Part model, mm, in its own coordinate system. Give positions to 0.01 mm unless a question says otherwise; leave off trailing zeros. Write each loop counter-clockwise with the first axis right and the second up, starting at its lowest first coordinate (ties: lowest second). Pieces come first, ordered by that corner, then holes. Notation, with made-up numbers: (6, -36.75) - (35, -36.75) arc R21 cw to (35, -7.75) - close; hole circle Ø5 at (50.25, -3). An arc over 180 degrees is marked (long way). Answer as a JSON object with one key per item and string values. Group by question number.
```python
from build123d import *

# Parameters (mm, degrees)
SKETCH1_R           = 4.445
SKETCH1_W           = 3.175
SKETCH1_H           = 12.7
SKETCH1_H_2         = 3.175
SKETCH1_W_2         = 25.4
BOSS_EXTRUDE1_DEPTH = 3.175


with BuildPart() as part:
    # Sketch1 → Boss-Extrude1 (new body)
    with BuildSketch(Plane.XY):
        with BuildLine():
            ThreePointArc((-23.00901311, 85.870805957), (0, -88.9), (23.00901311, 85.870805957))
            add(Edge.make_bspline(
                [(23.00901311, 85.870805957), (14.830841114, 88.062140539), (8.89, 90.527472624), (8.89, 94.760805957)],
                knots=[0, 0, 0, 0, 1, 1, 1, 1], degree=3))
            ThreePointArc((8.89, 94.760805957), (0, 103.650805957), (-8.89, 94.760805957))
            add(Edge.make_bspline(
                [(-23.00901311, 85.870805957), (-14.830841114, 88.062140539), (-8.89, 90.527472624), (-8.89, 94.760805957)],
                knots=[0, 0, 0, 0, 1, 1, 1, 1], degree=3))
        make_face()
        with Locations((0, 94.760805957)):
            Circle(SKETCH1_R, mode=Mode.SUBTRACT)
        with Locations((77.7875, 25.38476)):
            Rectangle(SKETCH1_W, SKETCH1_H, mode=Mode.SUBTRACT)
        Rectangle(SKETCH1_W, SKETCH1_H_2, mode=Mode.SUBTRACT)
        with Locations((77.7875, -25.41524)):
            Rectangle(SKETCH1_W, SKETCH1_H, mode=Mode.SUBTRACT)
        with Locations((-77.7875, -25.41524)):
            Rectangle(SKETCH1_W, SKETCH1_H, mode=Mode.SUBTRACT)
        with Locations((-77.7875, 25.38476)):
            Rectangle(SKETCH1_W, SKETCH1_H, mode=Mode.SUBTRACT)
        with Locations((0, 80.9625)):
            Rectangle(SKETCH1_W_2, SKETCH1_H_2, mode=Mode.SUBTRACT)
        with Locations((0, -80.9625)):
            Rectangle(SKETCH1_W_2, SKETCH1_H_2, mode=Mode.SUBTRACT)
    extrude(amount=BOSS_EXTRUDE1_DEPTH)


solid = part.part
```
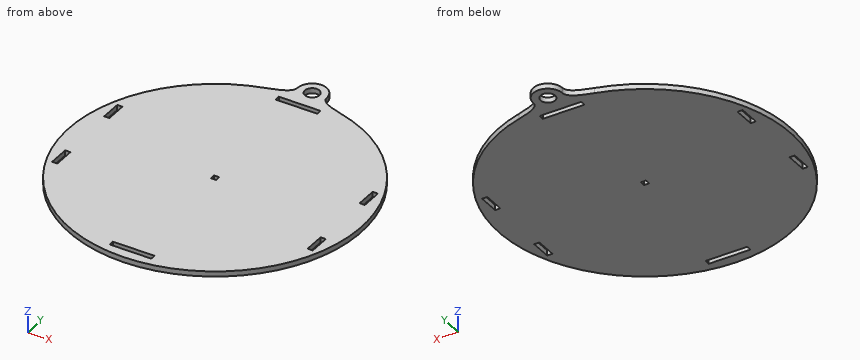
1) Band-saw the part on B-B (z = 1.15). State how many separate pieces and enclosed holes the cut face has, plus the area to 3 significant figures.
2) Drop flat-ended pins along their axis: P1, Ø1.6, axis at y = 81.5, z = 1.5, coming from the +X side; P2, Ø1, axis at y = 23, z = 1, coming from the -X side; P3, Ø1.5, axis at y = 46.5, z = 2.5, coming from the -X side. Give the stop position or say it passes through.
3) Probe line 1 (X direction, y = -19.5, z = 1.8) (3 decimals); line 2 (X direction, y = 26, z = 1.85) (3 decimals); line 3 (X direction, y = -33, z = 0.9). List the from-to ranges inside material, lowest first.
4) Band-saw the part on C-C (y = -46). List the corners of the cut face in (x, z) (3 decimals).
5) Band-saw the part on A-A (y = -24). List the corners of the cut face in (x, z) (3 decimals).
6) Band-saw the part on D-D (x = -43). List the corners of the cut face in (y, z) (3 decimals).
Verdict:
{
 "1": {"separate pieces": "1", "enclosed holes": "8", "area": "24,700 mm2"},
 "2": {"P1": "x = 37.29", "P2": "x = -86.01", "P3": "x = -76.22"},
 "3": {"line 1": "-86.735 to -79.375, -76.2 to 76.2, 79.375 to 86.735", "line 2": "-85.013 to -79.375, -76.2 to 76.2, 79.375 to 85.013", "line 3": "-82.55 to 82.55"},
 "4": {"outline": "(-76.074, 0) - (76.074, 0) - (76.074, 3.175) - (-76.074, 3.175) - close"},
 "5": {"outline": "(-85.599, 0) - (-79.375, 0) - (-79.375, 3.175) - (-85.599, 3.175) - close; (-76.2, 0) - (76.2, 0) - (76.2, 3.175) - (-76.2, 3.175) - close; (79.375, 0) - (85.599, 0) - (85.599, 3.175) - (79.375, 3.175) - close"},
 "6": {"outline": "(-77.809, 0) - (77.809, 0) - (77.809, 3.175) - (-77.809, 3.175) - close"}
}
